Could you check a few things on this model? Use its own coordinates, in mm. A direction names the side the tool comes from. Round coordinates to 2 decimals unless told otherwise and drop trailing zeros. Loops run counter-clockwise (first coordinate to the right, second up) from the corner with the lowest first, then second, coordinate; pieces in that order, holes last.
Autodesk Inventor part; units mm, degrees
ref_plane "YZ Plane" through (0, 0, 0) normal (1, 0, 0) x (0, 1, 0)
ref_plane "XZ Plane" through (0, 0, 0) normal (0, 1, 0) x (-1, 0, 0)
ref_plane "XY Plane" through (0, 0, 0) normal (0, 0, 1) x (1, 0, 0)
sketch "Skizze1" plane through (0, 0, 0) normal (0, 1, 0) x (-1, 0, 0)
  line L0 (0, 0) -> (188, 0)
  line L1 (188, 0) -> (188, -400)
  line L2 (188, -400) -> (0, -400)
  line L3 (0, -400) -> (0, 0)
  dimension "d1" = 188
  dimension "d2" = 400
extrude "Extrusion1" add sketch "Skizze1" along normal blind 15
sketch "Skizze2" plane through (0, 15, 0) normal (0, 1, 0) x (1, 0, 0)
  line L0 (-173, 15) -> (-155, 15)
  line L1 (-155, 15) -> (-155, 385)
  line L2 (-155, 385) -> (-173, 385)
  line L3 (-173, 385) -> (-173, 15)
  line L4 (-43, 15) -> (-61, 15)
  line L5 (-61, 15) -> (-61, 150)
  line L6 (-61, 150) -> (-43, 150)
  line L7 (-43, 150) -> (-43, 15)
  line L8 (-43, 385) -> (-61, 385)
  line L9 (-61, 385) -> (-61, 250)
  line L10 (-61, 250) -> (-43, 250)
  line L11 (-43, 250) -> (-43, 385)
  line L12 (-188, 0) -> (0, 0)
  line L13 (0, 0) -> (0, 400)
  dimension "d5" = 18
  dimension "d6" = 370
  dimension "d7" = 18
  dimension "d8" = 135
  dimension "d9" = 135
  dimension "d10" = 18
  dimension "d11" = 15
  dimension "d12" = 150
  dimension "d13" = 250
  dimension "d14" = 43
  dimension "d15" = 155
  dimension "d16" = 43
extrude "Extrusion2" add sketch "Skizze2" along normal blind 15
sketch "Skizze3" plane through (0, 30, 0) normal (0, 1, 0) x (1, 0, 0)
  point P0 (0, 0)
  point P1 (-52, 45)
  point P2 (-52, 120)
  point P3 (-52, 280)
  point P4 (-52, 355)
  point P5 (-164, 355)
  point P6 (-164, 200)
  point P7 (-164, 45)
hole "Bohrung1" at (-52, 30, -45) at (-52, 30, -120) at (-52, 30, -280) at (-52, 30, -355) at (-164, 30, -355) at (-164, 30, -200) at (-164, 30, -45) direction (0, -1, 0) diameter 4.5 depth 25 tip angle 118 countersink diameter 9 countersink angle 90
sketch "Skizze4" plane through (0, 0, 0) normal (0, -1, 0) x (1, 0, 0)
  line L0 (0, 0) -> (-188, 0)
  line L1 (0, -400) -> (0, 0)
  point P0 (-23, -200)
  point P1 (-23, -100)
  point P2 (-23, -300)
  dimension "d26" = 100
  dimension "d27" = 200
  dimension "d28" = 300
  dimension "d29" = 23
  dimension "d30" = 23
  dimension "d31" = 23
hole "Bohrung2" at (-23, 0, -100) at (-23, 0, -200) at (-23, 0, -300) direction (0, 1, 0) diameter 6.5 end through all countersink diameter 11.3 countersink angle 90
chamfer "Fase1" distance 2 angle 45 6 edges at (-188, 0, -200) (-94, 0, 0) (-188, 7.5, 0) (0, 0, -200) (-94, 0, -400) (-188, 7.5, -400)
properties part number "frontHolz" material "Pappel"
Item 1: If we section it at C-C, the plane z = -72: Please give me the cut outline in (x, y).
Results list:
outline: (-188, 2) - (-186, 0) - (-2, 0) - (0, 2) - (0, 15) - (-43, 15) - (-43, 30) - (-61, 30) - (-61, 15) - (-155, 15) - (-155, 30) - (-173, 30) - (-173, 15) - (-188, 15) - close
Item 2: For faces 4 (the flat face through (-61, 22, -82)), 5 (the flat face through (-43, 22, -317)), 6 (the flat face through (-164, 22, -15)), 7 (the flat face through (-52, 22, -385)), which set-ups out of +Z, -Z, +X, -X, +Y, -Y let a thin tool reach every point of the face, with its end or its side?
Results list:
face 4: +Z, -Z, +Y
face 5: +Z, -Z, +X, +Y
face 6: +Z, +X, -X, +Y
face 7: -Z, +X, -X, +Y
Item 3: We'd pull the mould along X, two halves only. Please class faces 1 (the flat face through (-52, 22, -150)), 2 (the conical face through (-163.28, 27.89, -197.72)), 3 (the flat face through (-43, 22, -83)): released by +X, released by -X, zero draft, split by the parting line, or undercut.
Results list:
face 1: zero draft
face 2: undercut
face 3: released by +X
Item 4: Will these pins go through, and if not, where does the flat tip stop? pin 1 (6 mm diameter, centred on x = -149.5, z = -101, fed in from +Y); pin 2 (6 mm diameter, centred on x = -164, z = -200, fed in from +Y); pin 3 (7.5 mm diameter, centred on y = 21, z = -205, fed in from +X).
Results list:
pin 1: stops at y = 15
pin 2: stops at y = 28.5
pin 3: stops at x = -155
Item 5: If I drill on line 1 along Z through (x, y) = (-52, 16.75); line 2 along Z through (x, y) = (-52, 11.25); line 3 along Z through (x, y) = (-57.5, 27), over which ranges is the centre line in solid material (lowest first)?
Results list:
line 1: z = -385 to -357.25, -352.75 to -282.25, -277.75 to -250, -150 to -122.25, -117.75 to -47.25, -42.75 to -15
line 2: z = -400 to -357.25, -352.75 to -282.25, -277.75 to -122.25, -117.75 to -47.25, -42.75 to 0
line 3: z = -385 to -250, -150 to -15
Item 6: If we section it at A-A, the plane z = -154: Please give me the cut outline in (x, y).
Results list:
outline: (-188, 2) - (-186, 0) - (-2, 0) - (0, 2) - (0, 15) - (-155, 15) - (-155, 30) - (-173, 30) - (-173, 15) - (-188, 15) - close
Item 7: If we section it at B-B, the plane x = -79.5: Please give me the cut outline in (y, z), then the cut area to 3 significant figures.
Results list:
outline: (0, -398) - (2, -400) - (15, -400) - (15, 0) - (2, 0) - (0, -2) - close
area: 6,000 mm2
